Input: dimensioned drawing with shaded views. Units: mm. Origin: part minimum x, y, z. A direction names the side the tool comes from. Coordinates: 2 decimals unless noted, no trailing zeros. Loops run counter-clockwise (first coordinate to the right, second up) from the corner with the lowest first, then second, coordinate; pieces in that order, holes last. Notation, with made-up numbers: (29.25, 51.5) - (77.25, 51.5) arc R30 cw to (77.25, 76.5) - close; hole circle Ø10 at (56.25, 42.25). An arc over 180 degrees is marked (long way). Use one line per item in the form item = value. Start each with the question number.
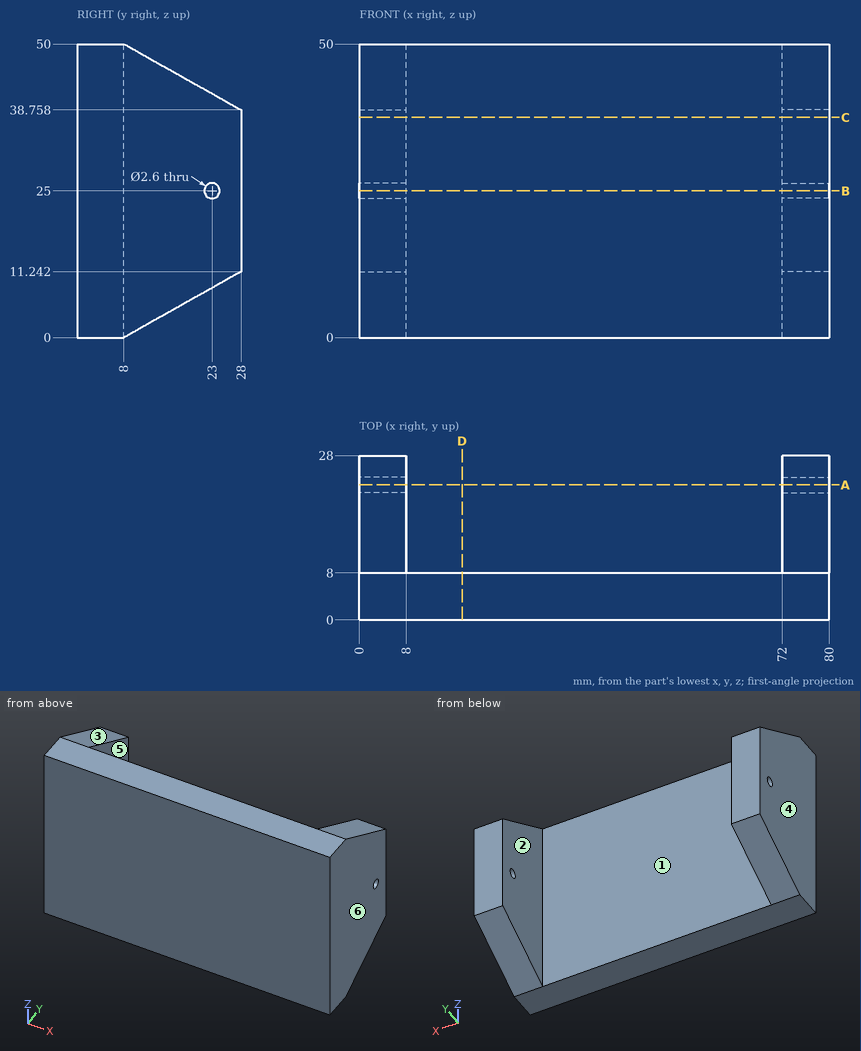
(1) Contact query for flat-ended pins moving along their axis: pin 1 (3 mm diameter, centred on y = 18.5, z = 21, fed in from -X); pin 2 (2.5 mm diameter, centred on y = 23, z = 25, fed in from -X); pin 3 (8 mm diameter, centred on x = 33, z = 36.5, fed in from +Y). Output: stop coordinate, or through.
(2) Cut plane C-C, the plane z = 37.5. Output: boundary loops of the cut face in (x, y).
(3) Mould query, pull axis X, two halves, no side actions, for the marked faces 1, 2, 3 and 4. Classes: +X half, -X half, draft (parallel to the pull), parting line (faces both ways), or undercut.
(4) Access query for the marked faces 5 and 6. Directions: +Z, -Z, +X, -X, +Y, -Y. A direction counts if a zero-diameter tool reaches every point of the face in a straight line with its end or side. Return the directions, or none.
(5) Cut plane A-A, the plane y = 23. Output: boundary loops of the cut face in (x, z).
(6) Cut plane B-B, the plane z = 25. Output: boundary loops of the cut face in (x, y).
(7) Cut plane D-D, the plane x = 17.5. Output: boundary loops of the cut face in (y, z), plus the area to 3 significant figures.
(8) Material intervals for line 1 (X direction, y = 15.5, z = 39); line 2 (Y direction, x = 5.5, z = 25); line 3 (Y direction, x = 35.5, z = 36), sorted ascending.
Recorded:
q1.pin_1 = 0
q1.pin_2 = through
q1.pin_3 = 8
q2.outline = (0, 0) - (80, 0) - (80, 28) - (72, 28) - (72, 8) - (8, 8) - (8, 28) - (0, 28) - close
q3.face_1 = undercut
q3.face_2 = undercut
q3.face_3 = draft
q3.face_4 = -X half
q4.face_5 = +Z, -Z, +Y
q4.face_6 = +Z, -Z, +X, +Y, -Y
q5.outline = (0, 8.43) - (8, 8.43) - (8, 23.7) - (0, 23.7) - close; (0, 26.3) - (8, 26.3) - (8, 41.57) - (0, 41.57) - close; (72, 8.43) - (80, 8.43) - (80, 23.7) - (72, 23.7) - close; (72, 26.3) - (80, 26.3) - (80, 41.57) - (72, 41.57) - close
q6.outline = (0, 0) - (80, 0) - (80, 21.7) - (72, 21.7) - (72, 8) - (8, 8) - (8, 21.7) - (0, 21.7) - close; (0, 24.3) - (8, 24.3) - (8, 28) - (0, 28) - close; (72, 24.3) - (80, 24.3) - (80, 28) - (72, 28) - close
q7.outline = (0, 0) - (8, 0) - (8, 50) - (0, 50) - close
q7.area = 400 mm²
q8.line_1 = 0 to 8, 72 to 80
q8.line_2 = 0 to 21.7, 24.3 to 28
q8.line_3 = 0 to 8
